Read the model definition and answer for the solid it produces. Units are mm, in the model's axes. A direction names the side the tool comes from. Round coordinates to 2 decimals unless told otherwise and drop trailing zeros. Write each loop counter-clockwise with the first axis right and the second up, starting at its lowest first coordinate (ties: lowest second). Pieces come first, ordered by that corner, then holes. Notation, with made-up numbers: (24.5, -13) -> (50.5, -13) arc R19 cw to (50.5, 5) -> close; hole circle Ø1 at (-26, -31). An arc over 180 degrees is marked (long way). Return JSON: item names as keys, results as strings. Group by question number.
(1) A cutting plane is placed at A-A on x = 0. Give the vertices of the cut face in (y, z).
(2) For faces 1 (the flat face through (0, 0, 19.05)), 2 (the flat face through (-3, 6, 0)), determine the directions among +Z, -Z, +X, -X, +Y, -Y from which every point of the face is accessible in a straight line to the end or side of a thin tool.
(3) A cutting plane is placed at D-D on z = -121. Give the vertices of the cut face in (x, y).
(4) Straight lines are drawn through the part: line 1 (Z direction, x = 3.75, y = 7.5); line 2 (Z direction, x = -0.5, y = -7); line 3 (X direction, y = -0.5, z = -107). For each, find the intervals that lie inside material, in ascending order.
(5) A cutting plane is placed at C-C on z = -65.5. Give the vertices of the cut face in (x, y), then the cut area to 3 significant figures.
(6) Given pin 1 (5 mm diameter, centred on y = -2, z = -94.5, fed in from -X); pin 2 (5 mm diameter, centred on x = -9, y = -4, fed in from +Z); pin 3 (4 mm diameter, centred on y = 3, z = -74.5, fed in from +X), each flat-ended and moving along its own axis, determine where each tip first touches the part or whether it passes through.
```python
from build123d import *

# Parameters (mm, degrees)
F0_R      = 6.35
F1_DEPTH  = 19.05
F2_R      = 7.62
F3_DEPTH  = 21.59
F5_R      = 8.89
F6_DEPTH  = 35.56
F8_R      = 10.16
F9_DEPTH  = 48.26
F11_R     = 11.682472
F12_DEPTH = 48.26


with BuildPart() as f1:
    # F0 (on Top) → F1 (new body)
    with BuildSketch(Plane.XY):
        Circle(F0_R)
    extrude(amount=F1_DEPTH)

    # F2 (on Top) → F3 (join)
    with BuildSketch(Plane.XY):
        Circle(F2_R)
    extrude(amount=-F3_DEPTH)

    # F5 (on offset) → F6 (join)
    with BuildSketch(Plane.XY.offset(-21.59)):
        Circle(F5_R)
    extrude(amount=-F6_DEPTH)

    # F8 (on offset) → F9 (join)
    with BuildSketch(Plane.XY.offset(-57.15)):
        Circle(F8_R)
    extrude(amount=-F9_DEPTH)

    # F11 (on offset) → F12 (join)
    with BuildSketch(Plane.XY.offset(-105.41)):
        Circle(F11_R)
    extrude(amount=-F12_DEPTH)


solid = f1.part
```
Checks:
{
 "1": {"outline": "(-11.68, -153.67) -> (11.68, -153.67) -> (11.68, -105.41) -> (10.16, -105.41) -> (10.16, -57.15) -> (8.89, -57.15) -> (8.89, -21.59) -> (7.62, -21.59) -> (7.62, 0) -> (6.35, 0) -> (6.35, 19.05) -> (-6.35, 19.05) -> (-6.35, 0) -> (-7.62, 0) -> (-7.62, -21.59) -> (-8.89, -21.59) -> (-8.89, -57.15) -> (-10.16, -57.15) -> (-10.16, -105.41) -> (-11.68, -105.41) -> close"},
 "2": {"face 1": "+Z, +X, -X, +Y, -Y", "face 2": "+Z"},
 "3": {"outline": "circle Ø23.36 at (0, 0)"},
 "4": {"line 1": "z = -153.67 to -21.59", "line 2": "z = -153.67 to 0", "line 3": "x = -11.67 to 11.67"},
 "5": {"outline": "circle Ø20.32 at (0, 0)", "area": "324 mm^2"},
 "6": {"pin 1": "stops at x = -10.16", "pin 2": "stops at z = 0", "pin 3": "stops at x = 10.11"}
}
